Input: part model. Units: mm. Frame: model coordinates. A direction names the side the tool comes from. Coordinates: 2 decimals unless noted, no trailing zeros. Loops run counter-clockwise (first coordinate to the right, second up) from the corner with the lowest first, then second, coordinate; pieces in that order, holes last. Notation, with made-up numbers: M 41.5,65.25 L 66.5,65.25 A6 ccw 66.5,72.25 Z; hole C 64.25,50 d6. An arc over 180 degrees is marked long. Use a Markdown table: item, result. Add a question column.
1. Section B-B on z = 0. Output: boundary loops of the cut face in (x, y).
2. Pin query (flat end, axial travel): pin 1 (1 mm diameter, centred on y = 5.5, z = 29.5, fed in from +X); pin 2 (15 mm diameter, centred on x = -76.5, z = 10, fed in from -Y); pin 3 (12 mm diameter, centred on y = 17, z = 12, fed in from -X); pin 4 (12 mm diameter, centred on x = -95.5, y = 13, fed in from -Z). Return the tip coordinate at first contact, or that it passes through.
3. Line query: L1, parallel to X at y = 28.5, z = -1; L2, parallel to Y at x = 8.5, z = 32; L3, parallel to Y at x = -34.5, z = 2.5. Output: solid intervals per line, ascending. Write a range as [from, to].
4. Section C-C on y = 6. Output: boundary loops of the cut face in (x, z).
5. Section A-A on x = -60. Output: boundary loops of the cut face in (y, z), then the cut area to 3 significant figures.
6. Set-up query: faces 1 (the flat face through (-147, 0, -27)), 2 (the flat face through (-308, 20, 8)), 3 (the flat face through (-148, 2, 0)). Return all of +Z, -Z, +X, -X, +Y, -Y with unobstructed straight access to the full face (end or side cutting, diameter ignored); none if empty.
7. Draft query along Z for faces 4 (the cylindrical face through (-9.76, 24.93, -2.17)), 5 (the flat face through (-148, 5, 40)), 6 (the cylindrical face through (24.994, 0.986, 0.55)). Return one class per face: +Z half, -Z half, draft (parallel to the pull), parting line (faces both ways), or undercut.
```python
from build123d import *

# Parameters (mm, degrees)
BOSS_EXTRUDE1_DEPTH = 10
SKETCH2_R           = 40
SKETCH2_R_2         = 30
BOSS_EXTRUDE2_DEPTH = 10
SKETCH3_R           = 10
BOSS_EXTRUDE3_DEPTH = 10
CUT_EXTRUDE1_DEPTH  = 2


with BuildPart() as part:
    # Sketch1 → Boss-Extrude1 (new body)
    with BuildSketch(Plane(origin=(0, 0, 0), x_dir=(1, 0, 0), z_dir=(0, 1, 0))):
        with BuildLine():
            Line((-300, 40), (0, 40))
            ThreePointArc((0, 40), (40, 0), (0, -40))
            Line((0, -40), (-300, -40))
            ThreePointArc((-300, -40), (-340, 0), (-300, 40))
        make_face()
    extrude(amount=BOSS_EXTRUDE1_DEPTH)

    # Sketch2 → Boss-Extrude2 (add)
    with BuildSketch(Plane(origin=(0, 10, 0), x_dir=(1, 0, 0), z_dir=(0, 1, 0))):
        with Locations(Location((-300, 0, 0), (0, 0, 270))):
            Circle(SKETCH2_R)
        with Locations(Location((0, 0, 0), (0, 0, 270))):
            Circle(SKETCH2_R_2)
    extrude(amount=BOSS_EXTRUDE2_DEPTH)

    # Sketch3 → Boss-Extrude3 (add)
    with BuildSketch(Plane(origin=(0, 20, 0), x_dir=(1, 0, 0), z_dir=(0, 1, 0))):
        with Locations(Location((0, 0, 0), (0, 0, 270))):
            Circle(SKETCH3_R)
        with Locations(Location((-300, 0, 0), (0, 0, 270))):
            Circle(SKETCH3_R)
    extrude(amount=BOSS_EXTRUDE3_DEPTH)

    # Sketch5 → Cut-Extrude1 (cut)
    with BuildSketch(Plane.XZ):
        with BuildLine():
            Line((-300, 25), (0, 25))
            ThreePointArc((0, 25), (25, 0), (0, -25))
            Line((0, -25), (-300, -25))
            ThreePointArc((-300, -25), (-325, 0), (-300, 25))
        make_face()
    extrude(amount=-CUT_EXTRUDE1_DEPTH, mode=Mode.SUBTRACT)


solid = part.part
```
Answers below:
| question | item | result |
|---|---|---|
| 1 | outline | M -340,0 L -325,0 L -325,2 L 25,2 L 25,0 L 40,0 L 40,10 L 30,10 L 30,20 L 10,20 L 10,30 L -10,30 L -10,20 L -30,20 L -30,10 L -260,10 L -260,20 L -290,20 L -290,30 L -310,30 L -310,20 L -340,20 Z |
| 2 | pin 1 | stops at x = 27.55 |
| 2 | pin 2 | stops at y = 2 |
| 2 | pin 3 | stops at x = -339.55 |
| 2 | pin 4 | stops at z = -40 |
| 3 | L1 | x = [-309.95, -290.05], [-9.95, 9.95] |
| 3 | L2 | y = [0, 10] |
| 3 | L3 | y = [2, 10] |
| 4 | outline | M -300,-40 L 0,-40 A40 ccw 0,40 L -300,40 A40 ccw Z |
| 5 | outline | M 0,-40 L 10,-40 L 10,40 L 0,40 L 0,25 L 2,25 L 2,-25 L 0,-25 Z |
| 5 | area | 700 mm² |
| 6 | face 1 | +Z, -Z, +X, -X, -Y |
| 6 | face 2 | +Y |
| 6 | face 3 | -Y |
| 7 | face 4 | parting line |
| 7 | face 5 | +Z half |
| 7 | face 6 | undercut |
